Could you check a few things on this model? Use its own coordinates, in mm. A direction names the side the tool comes from. Give positions to 0.01 mm unless a question says otherwise; leave off trailing zeros. Write each loop counter-clockwise with the first axis right and the second up, starting at its lowest first coordinate (ties: lowest second). Pieces come first, ordered by that corner, then holes. Notation, with made-up numbers: (-15.75, 51.5) -> (-8.75, 51.5) arc R8 ccw to (-8.75, 59.5) -> close; hole circle Ø5 at (81.5, 2). An arc over 180 degrees is marked (long way). Write item = value, one per line. Start each with the question number.
```python
from build123d import *

# Parameters (mm, degrees)
BOSS_EXTRUDE1_DEPTH = 5.55625
SKETCH2_R           = 2.6035
CUT_EXTRUDE1_DEPTH  = 27.356702141


with BuildPart() as part:
    # Sketch1 → Boss-Extrude1 (new, symmetric)
    with BuildSketch(Plane.XY):
        with BuildLine():
            Line((-21.2598, -8.2042), (0, -8.2042))
            ThreePointArc((0, -8.2042), (3.700135792, 7.322423968), (-6.604900662, -4.86664))
            Line((-6.604900662, -4.86664), (-5.112152215, -3.766749226))
            ThreePointArc((-5.112152215, -3.766749226), (2.863882192, 5.667510811), (0, -6.35))
            Line((0, -6.35), (-21.2598, -6.35))
            Line((-21.2598, -6.35), (-21.2598, -8.2042))
        make_face()
    extrude(amount=BOSS_EXTRUDE1_DEPTH, both=True)

    # Sketch2 → Cut-Extrude1 (cut, through all)
    with BuildSketch(Plane(origin=(0, -6.35, 0), x_dir=(1, 0, 0), z_dir=(0, 1, 0))):
        with Locations(Location((-16.0528, 0, 0), (0, 0, 270))):
            Circle(SKETCH2_R)
    extrude(amount=-CUT_EXTRUDE1_DEPTH, mode=Mode.SUBTRACT)


solid = part.part
```
(1) On a 3-axis mill with a long thin cutter (end or side, diameter ignored), from which of +Z, -Z, +X, -X, +Y, -Y can I reach the whole of each face in a straight line? I mean faces 1 (the flat face through (-11, -8.204, 0)), 2 (the flat face through (-10, -6.35, 0)), 3 (the flat face through (-5.869, -4.324, 0.078)). Say none if no direction works.
(2) Imagine slicing it at D-D (z = -3). Please give me the cut outline in (x, y), then the cut area to 3 significant figures.
(3) Imagine slicing it at A-A (y = 0). Please give me the cut outline in (x, z), then the cut area to 3 significant figures.
(4) I'm going to push flat-ended pins straight in: pin 1 (4.5 mm diameter, centred on x = -16.05, z = 0, fed in from +Y); pin 2 (4 mm diameter, centred on x = 3, z = 3, fed in from -Y); pin 3 (3.5 mm diameter, centred on x = -10, z = -1, fed in from +Y); pin 4 (2 mm diameter, centred on x = 1.5, z = -3, fed in from -Y). Where does each tip first touch, or does it pass through?
(5) We'd pull the mould along X, two halves only. Please class faces 4 (the flat face through (-7, -1, -5.556)), 5 (the flat face through (-21.26, -7, 0)), 6 (the cylindrical face through (3.97, 7.18, 0.08)), 7 (the cylindrical face through (-18.594, -7.264, -0.564)): released by +X, released by -X, zero draft, split by the parting line, or undercut.
(6) Imagine slicing it at C-C (x = -15.5). Please give me the cut outline in (y, z), then the cut area to 3 significant figures.
(7) If I drill on line 1 along X through (y, z) = (-0.25, 5); line 2 along Y through (x, z) = (-10.75, 2.5); line 3 along Y through (x, z) = (-3.75, 2.75), over which ranges is the centre line in solid material (lowest first)? Write a range as from..to.
(8) Imagine slicing it at B-B (z = 0). Please give me the cut outline in (x, y).
Answers below:
q1.face_1 = +Z, -Z, +X, -X, -Y
q1.face_2 = +Z, -Z, -X
q1.face_3 = +Z, -Z
q2.outline = (-21.26, -8.2) -> (0, -8.2) arc R8.2 ccw (long way) to (-6.6, -4.87) -> (-5.11, -3.77) arc R6.35 cw (long way) to (0, -6.35) -> (-21.26, -6.35) -> close
q2.area = 112 mm^2
q3.outline = (-8.2, -5.56) -> (-6.35, -5.56) -> (-6.35, 5.56) -> (-8.2, 5.56) -> close; (6.35, -5.56) -> (8.2, -5.56) -> (8.2, 5.56) -> (6.35, 5.56) -> close
q3.area = 41.2 mm^2
q4.pin_1 = through
q4.pin_2 = -8.14
q4.pin_3 = -6.35
q4.pin_4 = -8.19
q5.face_4 = zero draft
q5.face_5 = released by -X
q5.face_6 = split by the parting line
q5.face_7 = undercut
q6.outline = (-8.2, -5.56) -> (-6.35, -5.56) -> (-6.35, -2.54) -> (-8.2, -2.54) -> close; (-8.2, 2.54) -> (-6.35, 2.54) -> (-6.35, 5.56) -> (-8.2, 5.56) -> close
q6.area = 11.2 mm^2
q7.line_1 = -8.2..-6.35, 6.35..8.2
q7.line_2 = -8.2..-6.35
q7.line_3 = -8.2..-6.35, 5.12..7.3
q8.outline = (-21.26, -8.2) -> (-18.66, -8.2) -> (-18.66, -6.35) -> (-21.26, -6.35) -> close; (-13.45, -8.2) -> (0, -8.2) arc R8.2 ccw (long way) to (-6.6, -4.87) -> (-5.11, -3.77) arc R6.35 cw (long way) to (0, -6.35) -> (-13.45, -6.35) -> close
